Autodesk Inventor part; units mm, degrees
ref_plane "YZ Plane" through (0, 0, 0) normal (1, 0, 0) x (0, 1, 0)
ref_plane "XZ Plane" through (0, 0, 0) normal (0, 1, 0) x (-1, 0, 0)
ref_plane "XY Plane" through (0, 0, 0) normal (0, 0, 1) x (1, 0, 0)
sketch "Sketch1" plane through (0, 0, 0) normal (0, 0, 1) x (1, 0, 0)
  line L0 (-15.875, 0) -> (-12.7, 0)
  line L1 (-12.7, 0) -> (-12.7, 22.352)
  line L2 (-9.525, 25.527) -> (9.525, 25.527)
  line L3 (12.7, 22.352) -> (12.7, 0)
  line L4 (12.7, 0) -> (15.875, 0)
  line L5 (15.875, 0) -> (15.875, 25.527)
  line L6 (12.7, 28.702) -> (-12.7, 28.702)
  line L7 (-15.875, 25.527) -> (-15.875, 0)
  arc A0 (-9.525, 25.527) -> (-12.7, 22.352) centre (-9.525, 22.352) ccw
  arc A1 (12.7, 22.352) -> (9.525, 25.527) centre (9.525, 22.352) ccw
  arc A2 (-12.7, 28.702) -> (-15.875, 25.527) centre (-12.7, 25.527) ccw
  arc A3 (15.875, 25.527) -> (12.7, 28.702) centre (12.7, 25.527) ccw
  line L8 (0, 35.2315) -> (0, -5.8719)
  point P0 (0, 0)
  dimension "d0" = 28.702
  dimension "d1" = 31.75
  dimension "d2" = 3.175
  dimension "d3" = 3.175
  dimension "d4" = 3.175
extrude "Extrusion1" add sketch "Sketch1" along normal mid plane 584.2
sketch "Sketch4" plane through (15.875, 0, 292.1) normal (1, 0, 0) x (0, 0, -1)
  line L0 (292.1, -5.7404) -> (292.1, 34.4424) construction
  line L1 (-116.84, 0) -> (701.04, 0) construction
  circle A0 centre (292.1, 12.7) radius 3.175
  point P0 (292.1, 0)
  dimension "d34" = 12.7
  dimension "d35" = 0
  dimension "d36" = 6.35
extrude "Extrusion4" cut sketch "Sketch4" against normal up to surface (31.75 mm away)
pattern_linear "Rectangular Pattern3" count 15 spacing 25.4 along (0, 0, 1) count 15 spacing 25.4 along (0, 0, -1) of "Extrusion4"
equation "\"d5\" = SupportLength"
equation "\"SupportLength\" = 584.2"
properties part number "CornerChannel" material "Aluminum 6061"
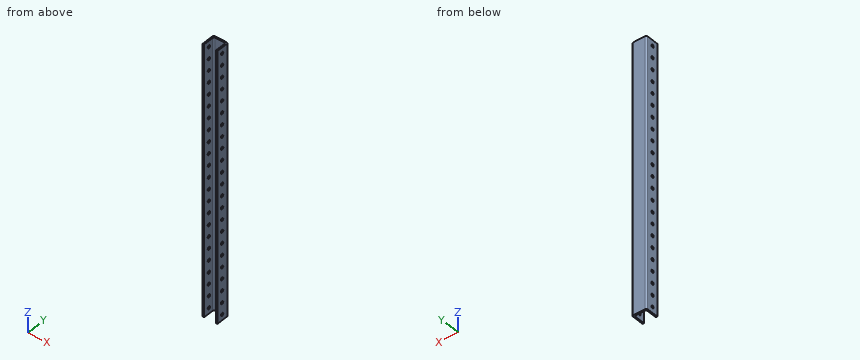
Work out the finished part from the listing and answer in its coordinate system (mm). Coordinates: 2 decimals unless noted, no trailing zeros. Loops run counter-clockwise (first coordinate to the right, second up) from the corner with the lowest first, then second, coordinate; pieces in that order, holes last. Notation, with made-up numbers: (-13, -32) -> (33, -32) arc R16 ccw to (33, -21) -> close; hole circle Ø7 at (8, -30.75). An arc over 180 degrees is marked (long way). Answer as CSV lines item,"result".
1) Straight lines are drawn through the part: probe 1 along X at (y, z) = (9, 42.5) (3 decimals); probe 2 along Y at (x, z) = (1, 117); probe 3 along X at (y, z) = (26.25, -244). For each, find the intervals that lie inside material, in ascending order.
A:
probe 1,"x = -15.875 to -12.7, 12.7 to 15.875"
probe 2,"y = 25.53 to 28.7"
probe 3,"x = -15.79 to 15.79"
2) The part is cut by section A-A (z = 34.5). Give the vertices of the cut face in (x, y) (3 decimals).
A:
outline,"(-15.875, 0) -> (-12.7, 0) -> (-12.7, 22.352) arc R3.175 cw to (-9.525, 25.527) -> (9.525, 25.527) arc R3.175 cw to (12.7, 22.352) -> (12.7, 0) -> (15.875, 0) -> (15.875, 25.527) arc R3.175 ccw to (12.7, 28.702) -> (-12.7, 28.702) arc R3.175 ccw to (-15.875, 25.527) -> close"
3) A flat-ended cylindrical pin translates along its axis: pin 1 (5 mm diameter, centred on x = 7, z = 20.5, fed in from -Y). Find the tip coordinate at first contact, or state that the pin passes through.
A:
pin 1,"stops at y = 25.53"
